from build123d import *

# Parameters (mm, degrees)
F0_R     = 0.55
F1_DEPTH = 0.15


with BuildPart() as f1:
    # F0 (on Top) → F1 (new body)
    with BuildSketch(Plane.XY):
        with BuildLine():
            Line((-2.709826, -0.125), (-0.688749, -0.125))
            ThreePointArc((-0.688749, -0.125), (0, -0.7), (0.688749, -0.125))
            Line((0.688749, -0.125), (17, -0.125))
            Line((17, -0.125), (17, 0.125))
            Line((17, 0.125), (0.688749, 0.125))
            ThreePointArc((0.688749, 0.125), (0, 0.7), (-0.688749, 0.125))
            Line((-0.688749, 0.125), (-2.709826, 0.125))
            ThreePointArc((-2.709826, 0.125), (-4.3, 0), (-2.709826, -0.125))
        make_face()
        with Locations((-3.5, 0)):
            Circle(F0_R, mode=Mode.SUBTRACT)
    extrude(amount=F1_DEPTH)


solid = f1.part
Read the model definition and answer for the solid it produces. Units are mm, in the model's axes. Round coordinates to 2 decimals unless told otherwise and drop trailing zeros. Write each loop counter-clockwise with the first axis right and the second up, starting at its lowest first coordinate (ties: lowest second). Pieces come first, ordered by that corner, then holes.
1. The part is cut by section D-D, the plane x = 13.75. Determine the outline of the cut face in (y, z) (3 decimals).
2. The part is cut by section C-C, the plane y = 0.35. Determine the outline of the cut face in (x, z), then the cut area to 3 significant figures.
3. The part is cut by section B-B, the plane z = 0.1. Determine the outline of the cut face in (x, y) (3 decimals).
4. The part is cut by section A-A, the plane x = -3.5. Determine the outline of the cut face in (y, z), then the cut area to 3 significant figures.
5. Given pin 1 Ø0.7 at (x, y) = (-3.5, 0) entering from +Z, flat-ended and moving along its own axis, determine where the tip first touches the part or whether it passes through.
6. Straight lines are drawn through the part: L1, parallel to X at y = -0.2, z = 0.1; L2, parallel to Y at x = -3.5, z = 0.05; L3, parallel to Y at x = 2.25, z = 0.1 (3 decimals). For each, find the intervals that lie inside material, in ascending order.
Values:
1. outline: (-0.125, 0) - (0.125, 0) - (0.125, 0.15) - (-0.125, 0.15) - close
2. outline: (-4.22, 0) - (-3.92, 0) - (-3.92, 0.15) - (-4.22, 0.15) - close; (-3.08, 0) - (-2.78, 0) - (-2.78, 0.15) - (-3.08, 0.15) - close; (-0.61, 0) - (0.61, 0) - (0.61, 0.15) - (-0.61, 0.15) - close
2. area: 0.270 mm2
3. outline: (-2.71, -0.125) - (-0.689, -0.125) arc R0.7 ccw to (0.689, -0.125) - (17, -0.125) - (17, 0.125) - (0.689, 0.125) arc R0.7 ccw to (-0.689, 0.125) - (-2.71, 0.125) arc R0.8 ccw (long way) to start; hole circle Ø1.1 at (-3.5, 0)
4. outline: (-0.8, 0) - (-0.55, 0) - (-0.55, 0.15) - (-0.8, 0.15) - close; (0.55, 0) - (0.8, 0) - (0.8, 0.15) - (0.55, 0.15) - close
4. area: 0.0750 mm2
5. pin 1: passes through
6. L1: x = -4.27 to -4.01, -2.99 to -2.73, -0.67 to 0.67
6. L2: y = -0.8 to -0.55, 0.55 to 0.8
6. L3: y = -0.125 to 0.125
